from build123d import *

# Parameters (mm, degrees)
PAD_DEPTH       = 5
PAD001_DEPTH    = 5
POCKET_DEPTH    = 5
SKETCH003_W     = 5
SKETCH003_H     = 1.5
POCKET001_DEPTH = 5
SKETCH004_R     = 2.5
POCKET002_DEPTH = 2
CHAMFER_SIZE    = 3
CHAMFER001_SIZE = 1


with BuildPart() as part:
    # Sketch → Pad (new body)
    with BuildSketch(Plane.XY):
        with BuildLine():
            ThreePointArc((2.5, 7.5), (0, 10), (-2.5, 7.5))
            Line((-2.5, 7.5), (-2.5, -7.5))
            ThreePointArc((-2.5, -7.5), (0, -10), (2.5, -7.5))
            Line((2.5, 7.5), (2.5, -7.5))
        make_face()
    extrude(amount=PAD_DEPTH)

    # Sketch001 (on Face6 of Pad) → Pad001 (join)
    with BuildSketch(Plane.XY.offset(5)):
        with BuildLine():
            ThreePointArc((5, 7.5), (0, 12.5), (-5, 7.5))
            Line((-5, 7.5), (-5, -7.5))
            ThreePointArc((-5, -7.5), (0, -12.5), (5, -7.5))
            Line((5, 7.5), (5, -7.5))
        make_face()
    extrude(amount=PAD001_DEPTH)

    # Sketch002 → Pocket (cut)
    with BuildSketch(Plane(origin=(0, 0, 0), x_dir=(1, 0, 0), z_dir=(0, 0, -1))):
        with BuildLine():
            ThreePointArc((2.5, 7.5), (0, 10), (-2.5, 7.5))
            Line((-2.5, 7.5), (-2.5, 4))
            ThreePointArc((-2.5, 4), (0, 1.5), (2.5, 4))
            Line((2.5, 7.5), (2.5, 4))
        make_face()
        with BuildLine():
            ThreePointArc((-2.5, -7.5), (0, -10), (2.5, -7.5))
            Line((2.5, -7.5), (2.5, -4))
            ThreePointArc((2.5, -4), (0, -1.5), (-2.5, -4))
            Line((-2.5, -7.5), (-2.5, -4))
        make_face()
    extrude(amount=-POCKET_DEPTH, mode=Mode.SUBTRACT)

    # Sketch003 (on Face10 of Pocket) → Pocket001 (cut)
    with BuildSketch(Plane(origin=(0, 0, 0), x_dir=(1, 0, 0), z_dir=(0, 0, -1))):
        with Locations((0, 3.25)):
            Rectangle(SKETCH003_W, SKETCH003_H)
    pocket001 = extrude(amount=-POCKET001_DEPTH, mode=Mode.SUBTRACT)

    # Mirrored: Pocket001 across XZ
    add(pocket001.mirror(Plane.XZ), mode=Mode.SUBTRACT)

    # Sketch004 (on Face6 of Mirrored) → Pocket002 (cut)
    with BuildSketch(Plane(origin=(0, 0, 5), x_dir=(1, 0, 0), z_dir=(0, 0, -1))):
        with Locations((0, -4)):
            Circle(SKETCH004_R)
        with Locations((0, 4)):
            Circle(SKETCH004_R)
    extrude(amount=-POCKET002_DEPTH, mode=Mode.SUBTRACT)

    # Chamfer
    chamfer_edges = [part.edges().sort_by_distance(p)[0] for p in [
        (0, -12.5, 10),
    ]]
    chamfer(chamfer_edges, length=CHAMFER_SIZE)

    # Chamfer001
    chamfer001_edges = [part.edges().sort_by_distance(p)[0] for p in [
        (0, -1.5, 0),
        (0, 1.5, 0),
    ]]
    chamfer(chamfer001_edges, length=CHAMFER001_SIZE)


solid = part.part
The listing builds one solid part. Answer for the finished solid, in the listing's coordinates (mm). A direction names the side the tool comes from. Round coordinates to 2 decimals unless told otherwise and drop trailing zeros. Write each loop counter-clockwise with the first axis right and the second up, starting at its lowest first coordinate (ties: lowest second). Pieces come first, ordered by that corner, then holes. Notation, with made-up numbers: M 22.25,38.5 L 58.25,38.5 A34 ccw 58.25,69.5 Z; hole C 68,81 d5. An arc over 180 degrees is marked long. Write each question's results on one line, items separated by ' | '. Start each with the question number.
Item 1: A cutting plane is placed at A-A on z = 1.25. Write down the section's boundary in (x, y), and give its area (3 significant figures).
Item 2: A cutting plane is placed at D-D on z = 9.75. Write down the section's boundary in (x, y).
Item 3: For faces 1 (the face through (2.5, 0, 2)), 2 (the face through (-2.5, 0, 2)), 3 (the face through (0, -4, 7)), 4 (the face through (-5, 0, 6)), determine the directions among +Z, -Z, +X, -X, +Y, -Y from which every point of the face is accessible in a straight line to the end or side of a thin tool.
Item 4: Flat-ended cylindrical pins translate along their axes: pin 1 Ø1.5 at (x, y) = (0, 7.5) entering from -Z; pin 2 Ø3 at (x, z) = (1.5, 8.5) entering from -Y; pin 3 Ø3 at (x, y) = (0, -4) entering from -Z. Find the tip coordinate at first contact, or state that the pin passes through.
Item 5: A cutting plane is placed at B-B on y = -4. Write down the section's boundary in (x, z), and give its area (3 significant figures).
Item 6: Straight lines are drawn through the part: L1, parallel to Y at x = 0, z = 6; L2, parallel to X at y = -4, z = 5.55; L3, parallel to Z at x = 1, y = -4.75. For each, find the intervals that lie inside material, in ascending order. Write a range as [from, to].
Item 7: For a pull along X with two mould halves and no side action, classify faces 5 (the face through (0, 1.2, 0.7)), 6 (the face through (0, 0, 10)), 7 (the face through (0.1, 12.5, 6)) as pulls with the +X half, pulls with the -X half, needs draft (parallel to the pull), parting line crosses it, or undercut.
Item 8: A cutting plane is placed at C-C on z = 5.75. Write down the section's boundary in (x, y), and give its area (3 significant figures).
Check sheet entries:
1) outline: M -2.5,-2.5 L -2,-2.5 A2.5 cw 2,-2.5 L 2.5,-2.5 L 2.5,2.5 L 2,2.5 A2.5 cw -2,2.5 L -2.5,2.5 Z | area: 19.4 mm²
2) outline: M -2.25,-7.5 A2.25 ccw 2.25,-7.5 L 2.25,7.5 A2.25 ccw -2.25,7.5 Z
3) face 1: -Z, +X, +Y, -Y | face 2: -Z, -X, +Y, -Y | face 3: -Z | face 4: +Z, -Z, -X, +Y, -Y
4) pin 1: z = 5 | pin 2: y = -12.32 | pin 3: z = 7
5) outline: M -5,5 L -2.5,5 L -2.5,7 L 2.5,7 L 2.5,5 L 5,5 L 5,7 L 2,10 L -2,10 L -5,7 Z | area: 31.0 mm²
6) L1: [-12.5, -6.5], [-1.5, 1.5], [6.5, 12.5] | L2: [-5, -2.5], [2.5, 5] | L3: [7, 10]
7) face 5: undercut | face 6: needs draft | face 7: parting line crosses it
8) outline: M -5,-7.5 A5 ccw 5,-7.5 L 5,7.5 A5 ccw -5,7.5 Z; hole C 0,-4 d5; hole C 0,4 d5 | area: 189 mm²
